from build123d import *

# Parameters (mm, degrees)
SKETCH3_R                  = 51.5
CUT_EXTRUDE1_DEPTH         = 185.176545738
SKETCH4_R                  = 4.2
CUT_EXTRUDE2_DEPTH         = 185.176545738
F_7_6_7_6_DIAMETER_HOLE1_D = 7.6
CIRPATTERN1_COUNT          = 16


with BuildPart() as part:
    # Sketch2 → Revolve1 (revolve)
    with BuildSketch(Plane(origin=(0, 0, 0), x_dir=(1, 0, 0), z_dir=(0, 1, 0)), mode=Mode.PRIVATE) as revolve1_sk:
        Polygon((0, 0), (0, 4.8), (-71, 4.8), (-85, 15.8), (-130, 15.8), (-130, 11), (-86.660142756, 11), (-72.660142756, 0), align=None)
    revolve(revolve1_sk.sketch.rotate(Axis((0, 0, 0), (0, 0, -1)), 180), axis=Axis((0, 0, 0), (0, 0, -1)))

    # Sketch3 → Cut-Extrude1 (cut, through all)
    with BuildSketch(Plane(origin=(0, 0, -4.8), x_dir=(-1, 0, 0), z_dir=(0, 0, -1))):
        Circle(SKETCH3_R)
    extrude(amount=-CUT_EXTRUDE1_DEPTH, mode=Mode.SUBTRACT)

    # Sketch4 → Cut-Extrude2 (cut, through all)
    with BuildSketch(Plane(origin=(0, 0, -4.8), x_dir=(-1, 0, 0), z_dir=(0, 0, -1))):
        with Locations((-10.071594305, -57.118849675)):
            Circle(SKETCH4_R)
        with Locations((-44.430577701, -37.281681362)):
            Circle(SKETCH4_R)
        with Locations((54.502172006, -19.837168313)):
            Circle(SKETCH4_R)
        with Locations((54.502172006, 19.837168313)):
            Circle(SKETCH4_R)
        with Locations((-10.071594305, 57.118849675)):
            Circle(SKETCH4_R)
        with Locations((-44.430577701, 37.281681362)):
            Circle(SKETCH4_R)
    extrude(amount=-CUT_EXTRUDE2_DEPTH, mode=Mode.SUBTRACT)

    # 7.6 _7.6_ Diameter Hole1 (through all)
    with Locations(Plane(origin=(0, 0, -15.8), x_dir=(-1, 0, 0), z_dir=(0, 0, -1))):
        with Locations((116.94592067, -20.620721098), (96.25, 0), (107.090930045, -9.369242345)):
            f_7_6_7_6_diameter_hole1 = Hole(F_7_6_7_6_DIAMETER_HOLE1_D / 2)

    # CirPattern1: 7.6 _7.6_ Diameter Hole1 ×16 about axis
    cirpattern1_axis = Axis((0, 0, 0), (0, 0, 1))
    for i in range(1, CIRPATTERN1_COUNT):
        add(f_7_6_7_6_diameter_hole1.rotate(cirpattern1_axis, i * 360 / CIRPATTERN1_COUNT), mode=Mode.SUBTRACT)


solid = part.part
Geometry check sheet. Reference: the model listing, model coordinates, mm. A direction names the side the tool comes from. Round coordinates to 2 decimals unless told otherwise and drop trailing zeros. One line per item, written item: value.
1. Mould release check, pull along X, two halves, no side actions. Record for faces 1 (the face through (85.123, 36.835, -13.366)), 2 (the face through (123.997, -39.048, -13.366)), 3 (the face through (112.15, -25.37, -13.37)), 4 (the face through (31, 85, -15.8)): released by +X, released by -X, zero draft, split by the parting line, or undercut.
The answers:
face 1: undercut
face 2: split by the parting line
face 3: undercut
face 4: zero draft
2. Set-up check for faces 5 (the face through (48, 21, -4.8)), 6 (the face through (-34.5, -99.41, -13.37)), 7 (the face through (85, 27, -11)): record each of +Z, -Z, +X, -X, +Y, -Y from which the full face is reachable in a straight line by a thin tool's end or side.
The answers:
face 5: -Z
face 6: +Z, -Z
face 7: +Z
3. Depth check by flat-ended pin: pin 1 Ø12 at (x, y) = (-82.35, 69.1) entering from +Z; pin 2 Ø1 at (y, z) = (-94, -12) entering from -X; pin 3 Ø4.5 at (x, y) = (82.35, -69.1) entering from +Z; pin 4 Ø11 at (x, y) = (-54.5, -19.84) entering from -Z. Enter the tip coordinate at first touch or a pass-through.
The answers:
pin 1: stops at z = -11
pin 2: stops at x = -90.32
pin 3: passes through
pin 4: stops at z = -4.8
4. Scan lines: L1, parallel to Z at x = 73, y = 97; L2, parallel to Y at x = 44, z = -14; L3, parallel to Y at x = -56, z = -9. Record each from-to range of solid material in increasing order.
The answers:
L1: z = -15.8 to -11
L2: y = -122.33 to -70.03, 70.03 to 122.33
L3: y = -62.76 to -51.89, 51.89 to 62.76
